Can you work these out from the model? Positions are in its coordinate system, mm. Give positions to 0.01 mm unless a question says otherwise; leave off trailing zeros. Write each loop counter-clockwise with the first axis right and the second up, starting at its lowest first coordinate (ties: lowest second). Pieces come first, ordered by that corner, then holes. Notation, with made-up numbers: (23, 81.5) -> (72, 81.5) arc R11 ccw to (72, 99.5) -> close; hole circle Ø3 at (43.25, 50.25). An arc over 180 degrees is marked (long way). Answer as CSV lines item,"result". Start each with the question number.
1. I'm going to push flat-ended pins straight in: P1, Ø1.8, axis at x = 15.5, z = -15.5, coming from the +Y side; P2, Ø1.5, axis at x = -1, z = 0.5, coming from the +Y side; P3, Ø1, axis at x = 24.5, y = -0.5, coming from the -Z side. Where does each tip first touch, or does it pass through?
2. I need wall thicknesses on line 1 (X direction, y = -1.2, z = -7.5); line 2 (Z direction, x = 15, y = -1.8); line 3 (X direction, y = -1.2, z = 30). Which ranges of each line are inside material? Lowest first, please. Write a range as [from, to].
3. If we section it at A-A on z = -13: Write out the boundary of the cut face in (x, y).
4. If we section it at C-C on x = -7.5: Write out the boundary of the cut face in (y, z), plus the area to 3 significant figures.
5. If we section it at D-D on y = -1.4: Count the separate pieces of the cut face and the enclosed holes in it, plus the area to 3 significant figures.
6. If we section it at B-B on z = 27: Write out the boundary of the cut face in (x, y).
Autodesk Inventor part; units mm, degrees
ref_plane "YZ Plane" through (0, 0, 0) normal (1, 0, 0) x (0, 1, 0)
ref_plane "XZ Plane" through (0, 0, 0) normal (0, 1, 0) x (-1, 0, 0)
ref_plane "XY Plane" through (0, 0, 0) normal (0, 0, 1) x (1, 0, 0)
sketch "Sketch1" plane through (0, 0, 0) normal (0, 1, 0) x (-1, 0, 0)
  line L0 (34.5, 34.5) -> (-34.5, 34.5)
  line L1 (-34.5, 34.5) -> (-34.5, -34.5)
  line L2 (-34.5, -34.5) -> (34.5, -34.5)
  line L3 (34.5, -34.5) -> (34.5, 34.5)
  point P0 (0, 0)
  point P1 (-34.5, 0)
  point P2 (0, 34.5)
  dimension "d0" = 69
extrude "Extrusion1" add sketch "Sketch1" against normal blind 2.5
sketch "Sketch2" plane through (0, -2.5, 0) normal (0, -1, 0) x (1, 0, 0)
  circle A0 centre (-15.5, 15.5) radius 19.9 construction
  line L0 (-15.5, 15.5) -> (15.5, -15.5) construction
  circle A1 centre (-15.5, 15.5) radius 1.5
  circle A2 centre (-11.5216, 30.0556) radius 1.5
  line L1 (-11.5216, 30.0556) -> (28.9823, 13.2551) construction
  arc A3 (26.633, 8.4441) -> (30.0556, 16.1214) centre (-11.5216, 30.0556) ccw construction
  arc A4 (27.9381, 7.7048) -> (31.4779, 15.6448) centre (-11.5216, 30.0556) ccw
  arc A5 (25.3278, 9.1834) -> (28.6334, 16.5981) centre (-11.5216, 30.0556) ccw
  arc A6 (31.4779, 15.6448) -> (28.6334, 16.5981) centre (30.0556, 16.1214) ccw
  arc A7 (25.3278, 9.1834) -> (27.9381, 7.7048) centre (26.633, 8.4441) ccw
  arc A8 (7.5557, 19.2499) -> (9.267, 23.0885) centre (-11.5216, 30.0556) ccw construction
  arc A9 (16.8524, 20.5464) -> (1.6817, 25.6307) centre (9.267, 23.0885) ccw
  arc A10 (0.5948, 23.1927) -> (14.5166, 15.3071) centre (7.5557, 19.2499) ccw
  arc A11 (14.5166, 15.3071) -> (16.8524, 20.5464) centre (-11.5216, 30.0556) ccw
  arc A12 (0.5948, 23.1927) -> (1.6817, 25.6307) centre (-11.5216, 30.0556) ccw
  circle A13 centre (7.5557, 19.2499) radius 18.25 construction
  line L2 (-11.5216, 31.5556) -> (-11.5216, 34.5) construction
  line L3 (34.5, 34.5) -> (-34.5, 34.5)
  line L4 (31.5556, 16.1214) -> (34.5, 16.1214) construction
  line L5 (34.5, -34.5) -> (34.5, 34.5)
  line L6 (0, 0) -> (7.5, 7.5) construction
  circle A14 centre (7.5, 7.5) radius 1.75
  line L7 (7.5178, 11.25) -> (7.5083, 9.25) construction
  line L8 (-34.5, 34.5) -> (-34.5, -34.5)
  arc A15 (-15.5, 34.5) -> (-34.5, 15.5) centre (-15.5, 15.5) ccw
  arc A16 (34.5, 15.5) -> (15.5, 34.5) centre (15.5, 15.5) ccw
  point P0 (8.7304, 21.6553)
  dimension "d5" = 3
  dimension "d18" = 3.5
  dimension "d3" = 39.8
  dimension "d4" = 3
  dimension "d6" = 43.85
  dimension "d7" = 7
  dimension "d8" = 4
  dimension "d10" = 7
  dimension "d11" = 4
  dimension "d12" = 16
  dimension "d13" = 36.5
  dimension "d14" = 25
  dimension "d15" = 15.5
  dimension "d16" = 15.5
  dimension "d17" = 7.5
  dimension "d19" = 2
extrude "Extrusion2" cut sketch "Sketch2" against normal through all
pattern_circular "Circular Pattern1" count 2 over 360 about axis through (0, -10, 0) along (0, 1, 0) of "Extrusion2"
properties part number "mount-plate_3DPrint"
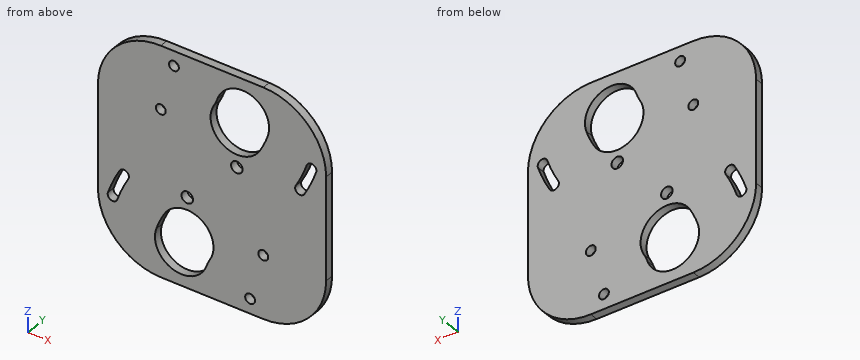
Computed values:
1,P1,"passes through"
1,P2,"stops at y = 0"
1,P3,"stops at z = -32.49"
2,line 1,"x = [-34.5, -27.8], [-25.47, -9.25], [-5.75, 34.5]"
2,line 2,"z = [-34.5, -16.91], [-14.09, 16.2], [28.67, 34.5]"
2,line 3,"x = [-27.78, -13.02], [-10.02, 5.24], [13.3, 27.78]"
3,outline,"(-34.5, -2.5) -> (-30.5, -2.5) -> (-30.5, 0) -> (-34.5, 0) -> close; (-27.24, -2.5) -> (-12.55, -2.5) -> (-12.55, 0) -> (-27.24, 0) -> close; (-2.56, -2.5) -> (34.5, -2.5) -> (34.5, 0) -> (-2.56, 0) -> close"
4,outline,"(-2.5, -34.5) -> (0, -34.5) -> (0, -30.89) -> (-2.5, -30.89) -> close; (-2.5, -11.25) -> (0, -11.25) -> (0, -9.25) -> (-2.5, -9.25) -> close; (-2.5, -5.75) -> (0, -5.75) -> (0, 34.5) -> (-2.5, 34.5) -> close"
4,area,"115 mm2"
5,separate pieces,"1"
5,enclosed holes,"10"
5,area,"3,800 mm2"
6,outline,"(-30.62, -2.5) -> (2.29, -2.5) -> (2.29, 0) -> (-30.62, 0) -> close; (16.25, -2.5) -> (30.62, -2.5) -> (30.62, 0) -> (16.25, 0) -> close"
